```python
from build123d import *

# Parameters (mm, degrees)
SKETCH1_W               = 200
SKETCH1_H               = 84
SKETCH1_R               = 2.25
SKETCH1_R_2             = 2.5
BOSS_EXTRUDE1_DEPTH     = 5
SKETCH2_W               = 200
SKETCH2_H               = 79
SKETCH2_R               = 2.25
BOSS_EXTRUDE2_DEPTH     = 3
CHAMFER1_SIZE           = 8
CHAMFER3_SIZE           = 3
SKETCH3_W               = 7.071067812
SKETCH3_H               = 2.6
CUT_EXTRUDE1_DEPTH      = 234.034075139
SKETCH4_R               = 2.5
CUT_EXTRUDE2_DEPTH      = 218.071416819
CUT_EXTRUDE3_DEPTH      = 218.071416819
CUT_EXTRUDE3_DEPTH_BACK = 218.071416819
SKETCH6_W               = 110
SKETCH6_H               = 35


with BuildPart() as part:
    # Sketch1 → Boss-Extrude1 (new body)
    with BuildSketch(Plane.XY):
        with Locations((100, 42)):
            Rectangle(SKETCH1_W, SKETCH1_H)
        with Locations((20, 9)):
            Circle(SKETCH1_R, mode=Mode.SUBTRACT)
        with Locations(Location((180, 9, 0), (0, 0, 180))):
            Circle(SKETCH1_R, mode=Mode.SUBTRACT)
        with Locations((20, 72)):
            Circle(SKETCH1_R, mode=Mode.SUBTRACT)
        with Locations(Location((180, 72, 0), (0, 0, 180))):
            Circle(SKETCH1_R, mode=Mode.SUBTRACT)
        with Locations((109.377508284, 51)):
            Circle(SKETCH1_R_2, mode=Mode.SUBTRACT)
        with Locations((129.377508284, 71)):
            Circle(SKETCH1_R_2, mode=Mode.SUBTRACT)
    extrude(amount=-BOSS_EXTRUDE1_DEPTH)

    # Sketch2 → Boss-Extrude2 (add)
    with BuildSketch(Plane(origin=(0, 0, -5), x_dir=(-1, 0, 0), z_dir=(0, 0, -1))):
        with Locations((-100, 44.5)):
            Rectangle(SKETCH2_W, SKETCH2_H)
        with Locations(Location((-20, 9, 0), (0, 0, 180))):
            Circle(SKETCH2_R, mode=Mode.SUBTRACT)
        with Locations((-180, 9)):
            Circle(SKETCH2_R, mode=Mode.SUBTRACT)
        with Locations(Location((-20, 72, 0), (0, 0, 180))):
            Circle(SKETCH2_R, mode=Mode.SUBTRACT)
        with Locations((-180, 72)):
            Circle(SKETCH2_R, mode=Mode.SUBTRACT)
    extrude(amount=BOSS_EXTRUDE2_DEPTH)

    # Chamfer1
    # the kernel refuses this chamfer: 8 mm, written as the material it takes off along each edge
    with BuildSketch(Plane(origin=(200, -15.573463904, -8), x_dir=(-0.9996219169112968, 0, -0.027495876610586296), z_dir=(0, 1, 0)), Plane(origin=(0, 104.573463904, -8), x_dir=(0.9996219169112968, 0, -0.027495876610586275), z_dir=(0, -1, 0))) as chamfer1_piece_1:
        Polygon((CHAMFER1_SIZE * 0.999621916911, CHAMFER1_SIZE * 0.0274958766106), (-CHAMFER1_SIZE * 0.0274958766106, CHAMFER1_SIZE * 0.999621916911), (0, 0), align=None)
    extrude(amount=120.146927807, mode=Mode.SUBTRACT)

    # Chamfer3
    chamfer3_edges = [part.edges().sort_by_distance(p)[0] for p in [
        (100, 84, -8),
    ]]
    chamfer(chamfer3_edges, length=CHAMFER3_SIZE)

    # Sketch3 → Cut-Extrude1 (cut, through all, along a direction that is not the sketch's normal)
    with BuildSketch(Plane(origin=(100, 0, -100), x_dir=(-0.7071067811865452, 0, -0.7071067811865498), z_dir=(0.7071067811865498, 0, -0.7071067811865452))):
        with Locations((-137.885822331, 1.3)):
            Rectangle(SKETCH3_W, SKETCH3_H)
    extrude(amount=-CUT_EXTRUDE1_DEPTH, dir=(1, 0, 0), mode=Mode.SUBTRACT)

    # Sketch4 → Cut-Extrude2 (cut, through all)
    with BuildSketch(Plane.XY):
        with Locations((129.377508284, 71)):
            Circle(SKETCH4_R)
        with Locations((109.377508284, 51)):
            Circle(SKETCH4_R)
    extrude(amount=-CUT_EXTRUDE2_DEPTH, mode=Mode.SUBTRACT)

    # Sketch6 → Cut-Extrude3 (cut, two sides: drawn at the far end of the back side and taken through both)
    with BuildSketch(Plane(origin=(0, 0, -8), x_dir=(-1, 0, 0), z_dir=(0, 0, -1)).offset(-CUT_EXTRUDE3_DEPTH_BACK)):
        with Locations((-100, 22.5)):
            Rectangle(SKETCH6_W, SKETCH6_H)
    extrude(amount=CUT_EXTRUDE3_DEPTH + CUT_EXTRUDE3_DEPTH_BACK, mode=Mode.SUBTRACT)


solid = part.part
```
Model file for the job. Use its own axes, mm. A direction names the side the tool comes from. Round coordinates to 2 decimals unless told otherwise and drop trailing zeros. Write each loop counter-clockwise with the first axis right and the second up, starting at its lowest first coordinate (ties: lowest second). Pieces come first, ordered by that corner, then holes. Notation, with made-up numbers: (-31.5, 86.5) -> (5.5, 86.5) arc R28 cw to (5.5, 125.5) -> close; hole circle Ø5 at (63, 20.5). An arc over 180 degrees is marked (long way). Answer as CSV lines item,"result".
1. Slice it at C-C, the plane x = 65. List the corners of the cut face in (y, z), plus the area to 4 significant figures.
Resolved:
outline,"(2.6, -5) -> (5, -5) -> (5, 0) -> (2.6, 0) -> close; (40, -8) -> (81, -8) -> (84, -5) -> (84, 0) -> (40, 0) -> close"
area,"359.5 mm²"
2. Slice it at D-D, the plane x = 20. List the corners of the cut face in (y, z), plus the area to 4 significant figures.
Resolved:
outline,"(2.6, -5) -> (5, -5) -> (5, -8) -> (6.75, -8) -> (6.75, 0) -> (2.6, 0) -> close; (11.25, -8) -> (69.75, -8) -> (69.75, 0) -> (11.25, 0) -> close; (74.25, -8) -> (81, -8) -> (84, -5) -> (84, 0) -> (74.25, 0) -> close"
area,"567.5 mm²"
3. Drill centre lines: line 1 (Y direction, x = 20, z = -2.8); line 2 (Y direction, x = 135, z = -2.75); line 3 (Y direction, x = 18, z = -4). Where is each one in solid material? Low to high.
Resolved:
line 1,"2.6 to 6.75, 11.25 to 69.75, 74.25 to 84"
line 2,"2.6 to 5, 40 to 84"
line 3,"2.6 to 7.97, 10.03 to 70.97, 73.03 to 84"
4. Slice it at A-A, the plane y = 28. List the corners of the cut face in (x, z).
Resolved:
outline,"(0, 0) -> (8, -8) -> (45, -8) -> (45, 0) -> close; (155, -8) -> (192, -8) -> (200, 0) -> (155, 0) -> close"
5. Slice it at B-B, the plane z = -3.5. List the corners of the cut face in (x, y), plus the area to 3 significant figures.
Resolved:
outline,"(3.5, 2.6) -> (196.5, 2.6) -> (196.5, 84) -> (3.5, 84) -> close; hole circle Ø4.5 at (20, 9); hole circle Ø4.5 at (20, 72); hole (45, 5) -> (155, 5) -> (155, 40) -> (45, 40) -> close; hole circle Ø5 at (109.38, 51); hole circle Ø5 at (129.38, 71); hole circle Ø4.5 at (180, 9); hole circle Ø4.5 at (180, 72)"
area,"11,800 mm²"
6. Tool access for faces 4 (the face through (4, 44, -4)), 5 (the face through (45, 22, -4)): list every direction of +Z, -Z, +X, -X, +Y, -Y with a clear straight run to the whole face (end or side of a thin tool).
Resolved:
face 4,"-Z, -X, +Y, -Y"
face 5,"+Z, -Z"
7. Pin check, flat tips, straight feed: pin 1 Ø10 at (x, y) = (36.5, 44) entering from +Z; pin 2 Ø3 at (y, z) = (74.5, -3) entering from +X; pin 3 Ø3 at (x, y) = (109.38, 51) entering from +Z; pin 4 Ø1.5 at (x, z) = (171.5, -7) entering from -Y. Stop position of each tip, or through.
Resolved:
pin 1,"z = 0"
pin 2,"x = 198.5"
pin 3,"through"
pin 4,"y = 5"
8. Mould opens along X. For faces 1 (the face through (155, 22, -4)), 2 (the face through (196, 43, -4)), 3 (the face through (97, 2.6, -4)) say: +X half, -X half, draft (parallel to the pull), parting line (faces both ways), or undercut.
Resolved:
face 1,"undercut"
face 2,"+X half"
face 3,"draft"
